Geometry: see drawing. Coordinates: mm, zero at the bounding-box minimum. A direction names the side the tool comes from. Give positions to 0.01 mm unless a question says otherwise; leave off trailing zeros. Order: outer loops, then holes, each group sorted by start corner. A loop starts at its lowest first (then second) coordinate and runs counter-clockwise, first axis right, second up. Notation, with made-up numbers: (-29.75, 19.25) -> (29.25, 19.25) arc R13 ccw to (29.25, 43.25) -> close; hole circle Ø6 at (-38.75, -23.75). An arc over 180 degrees is marked (long way). One line per item, written item: value. Start each with the question number.
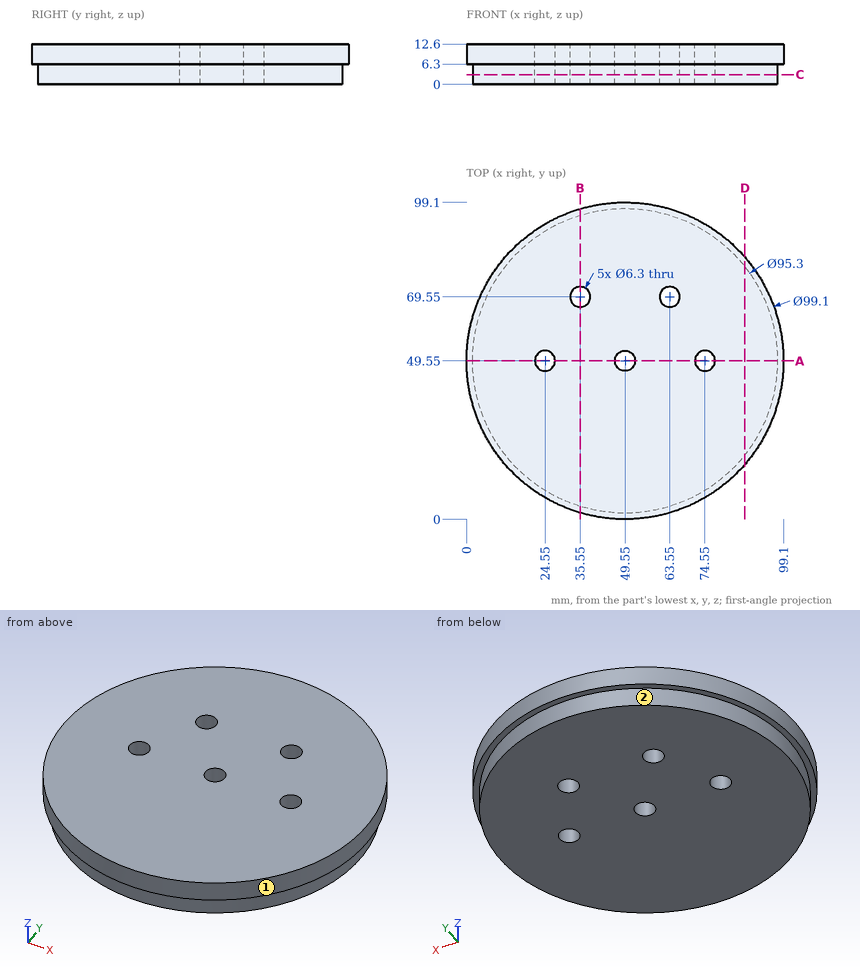
1. Pin query (flat end, axial travel): P1, Ø6, axis at x = 21.5, y = 50, coming from the -Z side; P2, Ø1, axis at x = 21.5, z = 2.5, coming from the +Y side; P3, Ø5, axis at x = 63.55, y = 69.55, coming from the +Z side; P4, Ø2, axis at x = 61, z = 10, coming from the +Y side. Return the tip coordinate at first contact, or that it passes through.
2. Cut plane B-B, the plane x = 35.55. Return loops of the section in (y, z).
3. Cut plane C-C, the plane z = 3. Return loops of the section in (x, y).
4. Access query for the marked faces 1 and 2. Directions: +Z, -Z, +X, -X, +Y, -Y. A direction counts if a zero-diameter tool reaches every point of the face in a straight line with its end or side. Return the directions, or none.
5. Cut plane D-D, the plane x = 87. Return loops of the section in (y, z).
6. Material intervals for L1, parallel to Y at x = 49.55, z = 8.75; L2, parallel to X at y = 68.5, z = 1.75; L3, parallel to X at y = 69.55, z = 7.75, sorted ascending. Write a range as [from, to].
7. Cut plane A-A, the plane y = 49.55. Return loops of the section in (x, z).
Answers follow:
1. P1: stops at z = 0
1. P2: stops at y = 88.43
1. P3: passes through
1. P4: stops at y = 97.99
2. outline: (2.02, 6.3) -> (4, 6.3) -> (4, 0) -> (66.4, 0) -> (66.4, 12.6) -> (2.02, 12.6) -> close; (72.7, 0) -> (95.1, 0) -> (95.1, 6.3) -> (97.08, 6.3) -> (97.08, 12.6) -> (72.7, 12.6) -> close
3. outline: circle Ø95.3 at (49.55, 49.55); hole circle Ø6.3 at (24.55, 49.55); hole circle Ø6.3 at (35.55, 69.55); hole circle Ø6.3 at (49.55, 49.55); hole circle Ø6.3 at (63.55, 69.55); hole circle Ø6.3 at (74.55, 49.55)
4. face 1: +Z, -Z
4. face 2: -Z
5. outline: (17.1, 6.3) -> (20.09, 6.3) -> (20.09, 0) -> (79.01, 0) -> (79.01, 6.3) -> (82, 6.3) -> (82, 12.6) -> (17.1, 12.6) -> close
6. L1: y = [0, 46.4], [52.7, 99.1]
6. L2: x = [5.83, 32.58], [38.52, 60.58], [66.52, 93.27]
6. L3: x = [4.22, 32.4], [38.7, 60.4], [66.7, 94.88]
7. outline: (0, 6.3) -> (1.9, 6.3) -> (1.9, 0) -> (21.4, 0) -> (21.4, 12.6) -> (0, 12.6) -> close; (27.7, 0) -> (46.4, 0) -> (46.4, 12.6) -> (27.7, 12.6) -> close; (52.7, 0) -> (71.4, 0) -> (71.4, 12.6) -> (52.7, 12.6) -> close; (77.7, 0) -> (97.2, 0) -> (97.2, 6.3) -> (99.1, 6.3) -> (99.1, 12.6) -> (77.7, 12.6) -> close
